```python
from build123d import *

# Parameters (mm, degrees)
ESBO_O1_W                = 26.7
ESBO_O1_H                = 39.3
RESSALTO_EXTRUS_O1_DEPTH = 38.5
CORTE_EXTRUS_O1_DEPTH    = 10
ESBO_O4_W                = 26.7
ESBO_O4_H                = 39.3
CORTE_EXTRUS_O2_DEPTH    = 10
ESBO_O5_W                = 26.7
ESBO_O5_H                = 39.3
ESBO_O5_W_2              = 22.6
ESBO_O5_H_2              = 27
CORTE_EXTRUS_O4_DEPTH    = 27
ESBO_O6_R                = 2.5
CORTE_EXTRUS_O5_DEPTH    = 5
ESBO_O7_W                = 2.05
ESBO_O7_H                = 1
RESSALTO_EXTRUS_O2_DEPTH = 4


with BuildPart() as part:
    # Esboço1 → Ressalto-extrusão1 (new body)
    with BuildSketch(Plane(origin=(0, 0, 0), x_dir=(1, 0, 0), z_dir=(0, 1, 0))):
        Rectangle(ESBO_O1_W, ESBO_O1_H)
    extrude(amount=-RESSALTO_EXTRUS_O1_DEPTH)

    # Esboço2 → Corte-extrusão1 (cut)
    with BuildSketch(Plane(origin=(0, 0, 0), x_dir=(1, 0, 0), z_dir=(0, 1, 0))):
        with BuildLine():
            Line((1.016622231, -18.102941176), (7.638740771, -11.999086257))
            ThreePointArc((7.638740771, -11.999086257), (8.829503459, -10.32964035), (9.25, -8.322615669))
            Line((9.25, -8.322615669), (9.25, 8.322615669))
            ThreePointArc((9.25, 8.322615669), (8.829503459, 10.32964035), (7.638740771, 11.999086257))
            Line((7.638740771, 11.999086257), (1.016622231, 18.102941176))
            ThreePointArc((1.016622231, 18.102941176), (0, 18.5), (-1.016622231, 18.102941176))
            Line((-1.016622231, 18.102941176), (-7.638740771, 11.999086257))
            ThreePointArc((-7.638740771, 11.999086257), (-8.829503459, 10.32964035), (-9.25, 8.322615669))
            Line((-9.25, 8.322615669), (-9.25, -8.322615669))
            ThreePointArc((-9.25, -8.322615669), (-8.829503459, -10.32964035), (-7.638740771, -11.999086257))
            Line((-7.638740771, -11.999086257), (-1.016622231, -18.102941176))
            ThreePointArc((-1.016622231, -18.102941176), (0, -18.5), (1.016622231, -18.102941176))
        make_face()
    extrude(amount=-CORTE_EXTRUS_O1_DEPTH, mode=Mode.SUBTRACT)

    # Esboço4 → Corte-extrusão2 (cut)
    with BuildSketch(Plane(origin=(0, 0, 0), x_dir=(1, 0, 0), z_dir=(0, 1, 0))):
        Rectangle(ESBO_O4_W, ESBO_O4_H)
        with BuildLine():
            ThreePointArc((-8.316488925, 12.734380374), (-9.74540415, 10.731045286), (-10.25, 8.322615669))
            Line((-10.25, 8.322615669), (-10.25, -8.322615669))
            ThreePointArc((-10.25, -8.322615669), (-9.74540415, -10.731045286), (-8.316488925, -12.734380374))
            Line((-8.316488925, -12.734380374), (-1.694370386, -18.838235294))
            ThreePointArc((-1.694370386, -18.838235294), (0, -19.5), (1.694370386, -18.838235294))
            Line((1.694370386, -18.838235294), (8.316488925, -12.734380374))
            ThreePointArc((8.316488925, -12.734380374), (9.74540415, -10.731045286), (10.25, -8.322615669))
            Line((10.25, -8.322615669), (10.25, 8.322615669))
            ThreePointArc((10.25, 8.322615669), (9.74540415, 10.731045286), (8.316488925, 12.734380374))
            Line((8.316488925, 12.734380374), (1.694370386, 18.838235294))
            ThreePointArc((1.694370386, 18.838235294), (0, 19.5), (-1.694370386, 18.838235294))
            Line((-1.694370386, 18.838235294), (-8.316488925, 12.734380374))
        make_face(mode=Mode.SUBTRACT)
    extrude(amount=-CORTE_EXTRUS_O2_DEPTH, mode=Mode.SUBTRACT)

    # Esboço5 → Corte-extrusão4 (cut)
    with BuildSketch(Plane.XZ.offset(38.5)):
        Rectangle(ESBO_O5_W, ESBO_O5_H)
        Rectangle(ESBO_O5_W_2, ESBO_O5_H_2, mode=Mode.SUBTRACT)
    extrude(amount=-CORTE_EXTRUS_O4_DEPTH, mode=Mode.SUBTRACT)

    # Esboço6 → Corte-extrusão5 (cut)
    with BuildSketch(Plane(origin=(0, -10, 0), x_dir=(1, 0, 0), z_dir=(0, 1, 0))):
        with Locations(Location((0, -9.5, 0), (0, 0, 270))):
            Circle(ESBO_O6_R)
        with Locations(Location((0, 9.5, 0), (0, 0, 270))):
            Circle(ESBO_O6_R)
        with Locations(Location((-3, 0, 0), (0, 0, 270))):
            Circle(ESBO_O6_R)
    extrude(amount=-CORTE_EXTRUS_O5_DEPTH, mode=Mode.SUBTRACT)

    # Esboço7 → Ressalto-extrusão2 (add)
    with BuildSketch(Plane.XZ.offset(11.5)):
        with Locations((12.325, 13)):
            Rectangle(ESBO_O7_W, ESBO_O7_H)
        with Locations((-12.325, 13)):
            Rectangle(ESBO_O7_W, ESBO_O7_H)
        with Locations((-12.325, -13)):
            Rectangle(ESBO_O7_W, ESBO_O7_H)
        with Locations((12.325, -13)):
            Rectangle(ESBO_O7_W, ESBO_O7_H)
    extrude(amount=RESSALTO_EXTRUS_O2_DEPTH)


solid = part.part
```
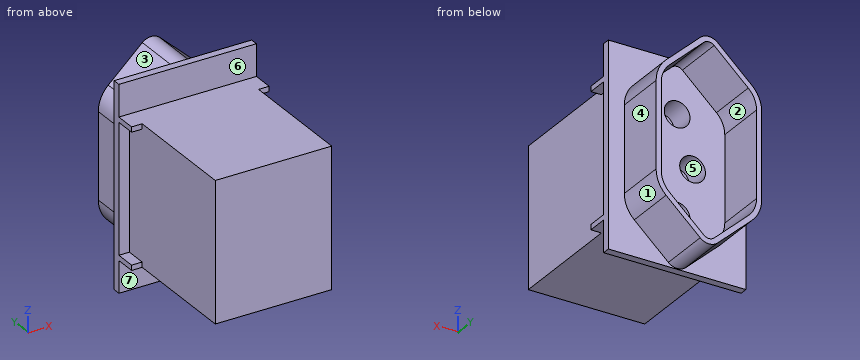
Input: part model. Units: mm. Frame: model coordinates. Face numbers are marked on the shaded views. A direction names the side the tool comes from. Round coordinates to 2 decimals unless told otherwise and drop trailing zeros. Loops run counter-clockwise (first coordinate to the right, second up) from the corner with the lowest first, then second, coordinate; pieces in that order, holes last. Notation, with made-up numbers: (41.25, -13) -> (77.25, -13) arc R5 ccw to (77.25, -8) -> close; hole circle Ø2 at (0.5, -11). An arc over 180 degrees is marked (long way). Use one line per item in the form item = value. Start each with the question number.
Item 1: Section query B-B on y = -14. Return the cut outline in (x, z), then the cut area to 3 significant figures.
Item 2: Contact query for flat-ended pins moving along their axis: pin 1 Ø0.8 at (x, z) = (12, 13) entering from -Y; pin 2 Ø3 at (y, z) = (-4, -1) entering from -X; pin 3 Ø1 at (x, y) = (12.5, -13.5) entering from +Z. Output: stop coordinate, or through.
Item 3: Section query C-C on x = 0. Return the cut outline in (y, z), then the cut area to 3 significant figures.
Item 4: Section query A-A on z = 0. Return the cut outline in (x, y).
Item 5: Material intervals for L1, parallel to X at y = -11.1, z = -9.5; L2, parallel to X at y = -13.7, z = 9.5; L3, parallel to Y at x = -3.25, z = 11.5, sorted ascending. Write a range as from..to.
Item 6: Mould query, pull axis X, two halves, no side actions, for the marked faces 1, 2 and 3. Classes: pulls with the +X half, pulls with the -X half, needs draft (parallel to the pull), parting line crosses it, or undercut.
Item 7: Set-up query: the marked faces 4, 5, 6 and 7. Return all of +Z, -Z, +X, -X, +Y, -Y with unobstructed straight access to the full face (end or side cutting, diameter ignored); none if empty.
Item 8: Section query D-D on y = -9. Return the cut outline in (x, z).
Ans:
q1.outline = (-13.35, -13.5) -> (13.35, -13.5) -> (13.35, -12.5) -> (11.3, -12.5) -> (11.3, 12.5) -> (13.35, 12.5) -> (13.35, 13.5) -> (-13.35, 13.5) -> (-13.35, 12.5) -> (-11.3, 12.5) -> (-11.3, -12.5) -> (-13.35, -12.5) -> close; hole circle Ø5 at (-3, 0); hole circle Ø5 at (0, -9.5); hole circle Ø5 at (0, 9.5)
q1.area = 559 mm^2
q2.pin_1 = -15.5
q2.pin_2 = -10.25
q2.pin_3 = 13.5
q3.outline = (-38.5, -13.5) -> (-11.5, -13.5) -> (-11.5, -19.65) -> (-10, -19.65) -> (-10, -19.5) -> (0, -19.5) -> (0, -18.5) -> (-10, -18.5) -> (-10, -12) -> (-15, -12) -> (-15, -7) -> (-10, -7) -> (-10, 7) -> (-15, 7) -> (-15, 12) -> (-10, 12) -> (-10, 18.5) -> (0, 18.5) -> (0, 19.5) -> (-10, 19.5) -> (-10, 19.65) -> (-11.5, 19.65) -> (-11.5, 13.5) -> (-38.5, 13.5) -> close
q3.area = 758 mm^2
q4.outline = (-13.35, -11.5) -> (-11.3, -11.5) -> (-11.3, -38.5) -> (11.3, -38.5) -> (11.3, -11.5) -> (13.35, -11.5) -> (13.35, -10) -> (10.25, -10) -> (10.25, 0) -> (9.25, 0) -> (9.25, -10) -> (-0.5, -10) -> (-0.5, -15) -> (-5.5, -15) -> (-5.5, -10) -> (-9.25, -10) -> (-9.25, 0) -> (-10.25, 0) -> (-10.25, -10) -> (-13.35, -10) -> close
q5.L1 = -13.35..-2.5, 2.5..13.35
q5.L2 = -11.3..-2.5, 2.5..11.3
q5.L3 = -38.5..-10
q6.face_1 = pulls with the +X half
q6.face_2 = undercut
q6.face_3 = pulls with the -X half
q7.face_4 = +Z, -Z, +X, +Y
q7.face_5 = +Y
q7.face_6 = +Z, +X, -X, -Y
q7.face_7 = -Z, +X, -X, -Y
q8.outline = (-10.25, -8.32) arc R6 ccw to (-8.32, -12.73) -> (-1.69, -18.84) arc R2.5 ccw to (1.69, -18.84) -> (8.32, -12.73) arc R6 ccw to (10.25, -8.32) -> (10.25, 8.32) arc R6 ccw to (8.32, 12.73) -> (1.69, 18.84) arc R2.5 ccw to (-1.69, 18.84) -> (-8.32, 12.73) arc R6 ccw to (-10.25, 8.32) -> close; hole (-9.25, -8.32) arc R5 ccw to (-7.64, -12) -> (-1.02, -18.1) arc R1.5 ccw to (1.02, -18.1) -> (7.64, -12) arc R5 ccw to (9.25, -8.32) -> (9.25, 8.32) arc R5 ccw to (7.64, 12) -> (1.02, 18.1) arc R1.5 ccw to (-1.02, 18.1) -> (-7.64, 12) arc R5 ccw to (-9.25, 8.32) -> close
